Could you check a few things on this drawing? It's one solid part, dimensions in mm from its lowest x, y, z. Coordinates: 2 decimals unless noted, no trailing zeros. Order: outer loops, then holes, each group sorted by start corner. A loop starts at its lowest first (then second) coordinate and runs counter-clockwise, first axis right, second up. Notation, with made-up numbers: (73.5, 46.25) - (110.5, 46.25) arc R28 cw to (110.5, 78.25) - close; hole circle Ø7 at (-18.75, 11). An arc over 180 degrees is marked (long way). Answer in a Markdown table with one row per item. Add a question column.
Item 1: If I drill on line 1 along X through (y, z) = (2.85, 12.5); line 2 along X through (y, z) = (2.9, 14.25) (1 decimal); line 3 along Z through (x, y) = (10.5, 2.9) (1 decimal), over which ranges is the centre line in solid material (lowest first)? Write a range as from..to.
Item 2: Will these pins go through, and if not, where does the flat tip stop? pin 1 Ø1.5 at (x, y) = (50.5, 2.5) entering from -Z; pin 2 Ø6 at (x, z) = (7.94, 12.7) entering from +Y.
Item 3: I want a section at C-C (x = 70). Please give me the cut outline in (y, z) (1 decimal).
Item 4: I want a section at B-B (y = 0.9). Count the separate pieces of the cut face and the enclosed holes in it, plus the area to 3 significant figures.
Item 5: I want a section at A-A (z = 12.7). Please give me the cut outline in (x, y) (1 decimal).
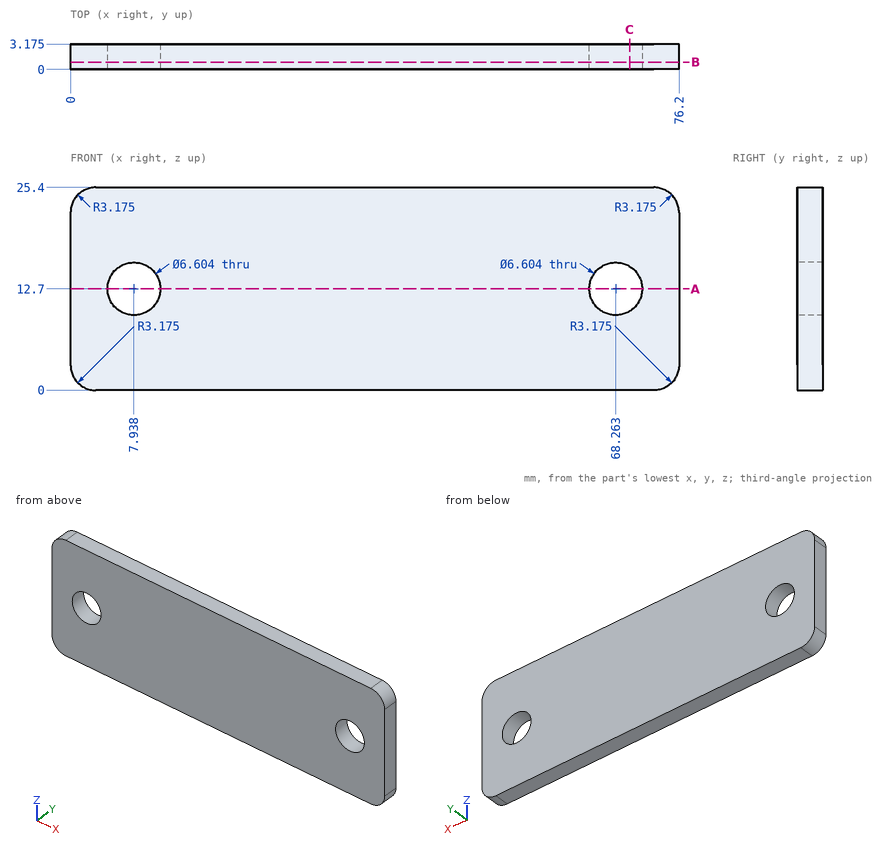
Values follow:
| question | item | result |
|---|---|---|
| 1 | line 1 | x = 0..4.64, 11.23..64.97, 71.56..76.2 |
| 1 | line 2 | x = 0..5, 10.9..65.3, 71.2..76.2 |
| 1 | line 3 | z = 0..10.6, 14.8..25.4 |
| 2 | pin 1 | stops at z = 0 |
| 2 | pin 2 | passes through |
| 3 | outline | (0, 0) - (3.2, 0) - (3.2, 9.9) - (0, 9.9) - close; (0, 15.5) - (3.2, 15.5) - (3.2, 25.4) - (0, 25.4) - close |
| 4 | separate pieces | 1 |
| 4 | enclosed holes | 2 |
| 4 | area | 1,860 mm^2 |
| 5 | outline | (0, 0) - (4.6, 0) - (4.6, 3.2) - (0, 3.2) - close; (11.2, 0) - (65, 0) - (65, 3.2) - (11.2, 3.2) - close; (71.6, 0) - (76.2, 0) - (76.2, 3.2) - (71.6, 3.2) - close |
